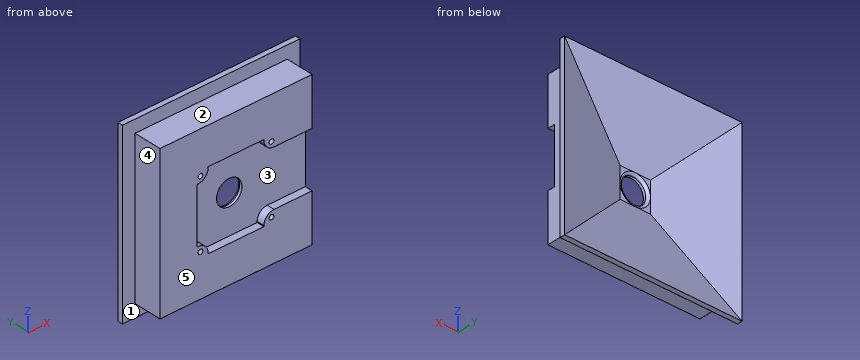
from build123d import *

# Parameters (mm, degrees)
SKETCH1_W            = 60
SKETCH1_H            = 60
BOSS_EXTRUDE1_DEPTH  = 6
SKETCH7_W            = 60
SKETCH7_H            = 60
SKETCH7_W_2          = 56
SKETCH7_H_2          = 56
BOSS_EXTRUDE4_DEPTH  = 7
SKETCH8_W            = 70
SKETCH8_H            = 70
SKETCH8_W_2          = 60
SKETCH8_H_2          = 60
BOSS_EXTRUDE5_DEPTH  = 2
SKETCH12_W           = 56
SKETCH12_H           = 56
BOSS_EXTRUDE10_DEPTH = 7
SKETCH13_W           = 12
SKETCH13_H           = 12
CUT_EXTRUDE3_DEPTH   = 8
SKETCH3_R            = 5
CUT_EXTRUDE4_DEPTH   = 52.17616649
SKETCH2_R            = 0.925
CUT_EXTRUDE5_DEPTH   = 3
SKETCH15_W           = 22
SKETCH15_H           = 4.335
SKETCH15_H_2         = 22
SKETCH15_R           = 5
SKETCH15_W_2         = 4.335
CUT_EXTRUDE6_DEPTH   = 3
SKETCH16_W           = 14.665
SKETCH16_H           = 22
CUT_EXTRUDE7_DEPTH   = 3
FILLET1_R            = 4
FILLET2_R            = 1


with BuildPart() as part:
    # Sketch1 → Boss-Extrude1 (new body)
    with BuildSketch(Plane(origin=(0, 0, 0), x_dir=(1, 0, 0), z_dir=(0, 1, 0))):
        Rectangle(SKETCH1_W, SKETCH1_H)
    extrude(amount=BOSS_EXTRUDE1_DEPTH)

    # Sketch7 → Boss-Extrude4 (add)
    with BuildSketch(Plane(origin=(0, 6, 0), x_dir=(1, 0, 0), z_dir=(0, 1, 0))):
        Rectangle(SKETCH7_W, SKETCH7_H)
        Rectangle(SKETCH7_W_2, SKETCH7_H_2, mode=Mode.SUBTRACT)
    extrude(amount=BOSS_EXTRUDE4_DEPTH)

    # Sketch8 → Boss-Extrude5 (add)
    with BuildSketch(Plane(origin=(0, 13, 0), x_dir=(1, 0, 0), z_dir=(0, 1, 0))):
        Rectangle(SKETCH8_W, SKETCH8_H)
        Rectangle(SKETCH8_W_2, SKETCH8_H_2, mode=Mode.SUBTRACT)
    extrude(amount=-BOSS_EXTRUDE5_DEPTH)

    # Sketch12 → Boss-Extrude10 (add)
    with BuildSketch(Plane(origin=(0, 6, 0), x_dir=(1, 0, 0), z_dir=(0, 1, 0))):
        Rectangle(SKETCH12_W, SKETCH12_H)
    extrude(amount=BOSS_EXTRUDE10_DEPTH)

    # Sketch13 → Cut-Extrude3 (cut)
    with BuildSketch(Plane(origin=(0, 13, 0), x_dir=(1, 0, 0), z_dir=(0, 1, 0))):
        Rectangle(SKETCH13_W, SKETCH13_H)
    extrude(amount=-CUT_EXTRUDE3_DEPTH, mode=Mode.SUBTRACT)

    # Sketch14 → section 1 of cut_loft1
    with BuildSketch(Plane(origin=(0, 13, 0), x_dir=(1, 0, 0), z_dir=(0, 1, 0)), mode=Mode.PRIVATE) as cut_loft1_s1:
        with BuildLine():
            Line((-35, 35), (-35, -35))
            Line((-35, -35), (35, -35))
            Line((35, -35), (35, 35))
            Line((35, 35), (-35, 35))
        make_face()
    # loft from a face of the part (cut_loft1)
    loft([part.faces().sort_by_distance((0, 5, 0))[0], cut_loft1_s1.sketch], mode=Mode.SUBTRACT)

    # Sketch3 → Cut-Extrude4 (cut, through all)
    with BuildSketch(Plane.XZ):
        with Locations(Location((0, 0, 0), (0, 0, 270))):
            Circle(SKETCH3_R)
    extrude(amount=-CUT_EXTRUDE4_DEPTH, mode=Mode.SUBTRACT)

    # Sketch2 → Cut-Extrude5 (cut)
    with BuildSketch(Plane.XZ):
        with Locations(Location((-14, -13.335, 0), (0, 0, 270))):
            Circle(SKETCH2_R)
        with Locations(Location((14, -13.335, 0), (0, 0, 270))):
            Circle(SKETCH2_R)
        with Locations(Location((14, 13.335, 0), (0, 0, 270))):
            Circle(SKETCH2_R)
        with Locations(Location((-14, 13.335, 0), (0, 0, 270))):
            Circle(SKETCH2_R)
    extrude(amount=-CUT_EXTRUDE5_DEPTH, mode=Mode.SUBTRACT)

    # Sketch15 → Cut-Extrude6 (cut)
    # profile 1 of 5: a face of its own
    with BuildSketch(Plane.XZ):
        with Locations((0, -13.1675)):
            Rectangle(SKETCH15_W, SKETCH15_H)
    # profile 2 of 5: a face of its own
    with BuildSketch(Plane.XZ):
        Rectangle(SKETCH15_W, SKETCH15_H_2)
        with Locations(Location((0, 0, 0), (0, 0, 270))):
            Circle(SKETCH15_R, mode=Mode.SUBTRACT)
    # profile 3 of 5: a face of its own
    with BuildSketch(Plane.XZ):
        with Locations((-13.1675, 0)):
            Rectangle(SKETCH15_W_2, SKETCH15_H_2)
    # profile 4 of 5: a face of its own
    with BuildSketch(Plane.XZ):
        with Locations((0, 13.1675)):
            Rectangle(SKETCH15_W, SKETCH15_H)
    # profile 5 of 5: a face of its own
    with BuildSketch(Plane.XZ):
        with Locations((13.1675, 0)):
            Rectangle(SKETCH15_W_2, SKETCH15_H_2)
    extrude(amount=-CUT_EXTRUDE6_DEPTH, mode=Mode.SUBTRACT)

    # Sketch16 → Cut-Extrude7 (cut)
    with BuildSketch(Plane.XZ):
        with Locations((22.6675, 0)):
            Rectangle(SKETCH16_W, SKETCH16_H)
    extrude(amount=-CUT_EXTRUDE7_DEPTH, mode=Mode.SUBTRACT)

    # Fillet1
    fillet1_edges = [part.edges().sort_by_distance(p)[0] for p in [
        (11, 1.5, -11),
        (-11, 1.5, -11),
        (-11, 1.5, 11),
        (11, 1.5, 11),
    ]]
    fillet(fillet1_edges, radius=FILLET1_R)

    # Fillet2
    fillet2_edges = [part.edges().sort_by_distance(p)[0] for p in [
        (0, 5, 5),
    ]]
    fillet(fillet2_edges, radius=FILLET2_R - 0.0001)  # a hair under: the kernel refuses the full size


solid = part.part
Input: part model. Units: mm. Frame: model coordinates. Face numbers are marked on the shaded views. A direction names the side the tool comes from. Coordinates: 2 decimals unless noted, no trailing zeros. Loops run counter-clockwise (first coordinate to the right, second up) from the corner with the lowest first, then second, coordinate; pieces in that order, holes last. Notation, with made-up numbers: (-4.75, 52) -> (14.25, 52) arc R16 cw to (14.25, 63) -> close; hole circle Ø6 at (3, -35.5). An arc over 180 degrees is marked (long way). Write each question's results on one line, items separated by ' | '. Start each with the question number.
Q1. Reachability of the marked faces 4 and 5 from +Z, -Z, +X, -X, +Y, -Y: full face, straight path, thin tool, end or side. Return the list, or none.
Q2. Pin query (flat end, axial travel): pin 1 (1 mm diameter, centred on y = 2, z = 25.5, fed in from -X); pin 2 (2.5 mm diameter, centred on x = 22.5, y = 2, fed in from -Z); pin 3 (3 mm diameter, centred on x = -19.5, z = 4.5, fed in from +Y). Return the tip coordinate at first contact, or that it passes through.
Q3. Ray query, line 1 (X direction, y = 3.7, z = 0); line 2 (Z direction, x = -10, y = 1.75) (3 decimals); line 3 (X direction, y = 1, z = 17). Return the intervals inside material, ascending. Write a range as from..to.
Q4. Section A-A, the plane y = 2. Return the cut outline in (x, z) (3 decimals).
Q5. Pull-direction query (Z, two-part tool) for the marked faces 1, 2 and 3; classes: released by +Z, released by -Z, zero draft, split by the parting line, or undercut.
Found:
1) face 4: +Z, -Z, -X, -Y | face 5: +Z, -Z, +X, -X, -Y
2) pin 1: x = -30 | pin 2: z = -30 | pin 3: y = 9.14
3) line 1: -30..-5, 5..30 | line 2: -30..-15.335, 15.335..30 | line 3: -30..30
4) outline: (-30, -30) -> (30, -30) -> (30, -11) -> (15, -11) arc R4 ccw to (11, -15) -> (11, -15.335) -> (-11, -15.335) -> (-11, -15) arc R4 ccw to (-15, -11) -> (-15.335, -11) -> (-15.335, 11) -> (-15, 11) arc R4 ccw to (-11, 15) -> (-11, 15.335) -> (11, 15.335) -> (11, 15) arc R4 ccw to (15, 11) -> (30, 11) -> (30, 30) -> (-30, 30) -> close; hole circle Ø1.85 at (-14, -13.335); hole circle Ø1.85 at (-14, 13.335); hole circle Ø1.85 at (14, -13.335); hole circle Ø1.85 at (14, 13.335)
5) face 1: zero draft | face 2: released by +Z | face 3: undercut
